Check sheet for the modelled part. Datum: model origin and axes. Units: mm. Give positions to 0.01 mm unless a question says otherwise; leave off trailing zeros. Order: outer loops, then holes, each group sorted by start corner. A loop starts at its lowest first (then second) coordinate and runs counter-clockwise, first axis right, second up.
Item 1: Gauge pin test, flat ends, axial feed: P1, Ø11, axis at x = 22.36, z = 13.1, coming from the -Y side; P2, Ø2, axis at x = -50, z = 9.6, coming from the +Y side; P3, Ø0.9, axis at x = 51, y = 2, coming from the +Z side; P4, Ø0.8, axis at y = 1, z = 22, coming from the -X side. Record the tip position at first contact, or that the pin passes through.
Item 2: Sectioned sample at A-A on x = 40.25. Record the boundary of the cut face in (y, z), and give its area (3 significant figures).
Item 3: Sectioned sample at C-C on z = 13.1. Count the separate pieces of the cut face and the enclosed holes in it, and give its area (4 significant figures).
Item 4: Sectioned sample at B-B on x = -50. Record the boundary of the cut face in (y, z), and give its area (3 significant figures).
Item 5: Material ranges on line 1 along Z through (x, y) = (-4.5, 1.65); line 2 along Z through (x, y) = (40.25, 2.25); line 3 along X through (y, z) = (1.15, 5.25), recorded low to high.
from build123d import *

# Parameters (mm, degrees)
SKETCH_1_R            = 3.5
SKETCH_1_W            = 10
SKETCH_1_H            = 3
EXTRUDE_1_DEPTH       = 3
HOLE_WIZARD_M31_D     = 3.4
HOLE_WIZARD_M31_DEPTH = 10
HOLE_WIZARD_M31_TIP   = 1.021463052
FILLET_1_R            = 0.5
FILLET_2_R            = 0.5


with BuildPart() as part:
    # Эскиз1 → Бобышка-Вытянуть1 (new body)
    with BuildSketch(Plane(origin=(0, 0, 0), x_dir=(1, 0, 0), z_dir=(0, 1, 0))):
        Polygon((-43.75, -21), (43.75, -21), (43.75, -18.5), (56.25, -18.5), (56.25, -15.5), (59.25, -15.5), (59.25, -5.5), (56.25, -5.5), (56.25, 0), (-56.25, 0), (-56.25, -5.5), (-59.25, -5.5), (-59.25, -15.5), (-56.25, -15.5), (-56.25, -18.5), (-43.75, -18.5), align=None)
        with Locations((-40.25, -13.1)):
            Circle(SKETCH_1_R, mode=Mode.SUBTRACT)
        with Locations((-31.305555556, -13.1)):
            Circle(SKETCH_1_R, mode=Mode.SUBTRACT)
        with Locations((-22.361111111, -13.1)):
            Circle(SKETCH_1_R, mode=Mode.SUBTRACT)
        with Locations((-13.416666667, -13.1)):
            Circle(SKETCH_1_R, mode=Mode.SUBTRACT)
        with Locations((-4.472222222, -13.1)):
            Circle(SKETCH_1_R, mode=Mode.SUBTRACT)
        with Locations((4.472222222, -13.1)):
            Circle(SKETCH_1_R, mode=Mode.SUBTRACT)
        with Locations((13.416666667, -13.1)):
            Circle(SKETCH_1_R, mode=Mode.SUBTRACT)
        with Locations((22.361111111, -13.1)):
            Circle(SKETCH_1_R, mode=Mode.SUBTRACT)
        with Locations((31.305555556, -13.1)):
            Circle(SKETCH_1_R, mode=Mode.SUBTRACT)
        with Locations((40.25, -13.1)):
            Circle(SKETCH_1_R, mode=Mode.SUBTRACT)
        with Locations((0, -22.5)):
            Rectangle(SKETCH_1_W, SKETCH_1_H)
    extrude(amount=EXTRUDE_1_DEPTH)

    # Отверстие с зазором M31
    with Locations(Plane(origin=(0, 3, 0), x_dir=(1, 0, 0), z_dir=(0, 1, 0))):
        with Locations((50, -9.6), (-50, -9.6)):
            Hole(HOLE_WIZARD_M31_D / 2, depth=HOLE_WIZARD_M31_DEPTH)
            with Locations((0, 0, -(HOLE_WIZARD_M31_DEPTH + HOLE_WIZARD_M31_TIP / 2))):  # 118° drill point
                Cone(0, HOLE_WIZARD_M31_D / 2, HOLE_WIZARD_M31_TIP, mode=Mode.SUBTRACT)

    # Скругление1
    fillet_1_edges = [part.edges().sort_by_distance(p)[0] for p in [
        (-59.25, 1.5, 15.5),
        (-59.25, 1.5, 5.5),
        (59.25, 1.5, 5.5),
        (59.25, 1.5, 15.5),
    ]]
    fillet(fillet_1_edges, radius=FILLET_1_R)

    # Скругление2
    fillet_2_edges = [part.edges().sort_by_distance(p)[0] for p in [
        (-56.25, 1.5, 18.5),
        (-56.25, 1.5, 0),
        (56.25, 1.5, 0),
        (56.25, 1.5, 18.5),
        (5, 1.5, 24),
        (-5, 1.5, 24),
    ]]
    fillet(fillet_2_edges, radius=FILLET_2_R)


solid = part.part
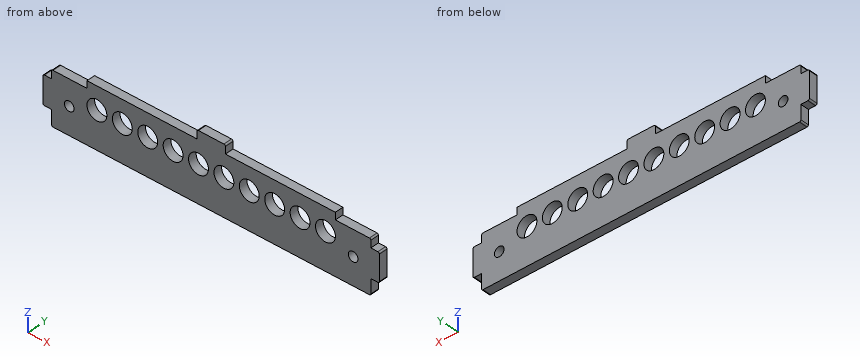
Report:
1. P1: stops at y = 0
1. P2: passes through
1. P3: stops at z = 18.5
1. P4: stops at x = -5
2. outline: (0, 0) - (3, 0) - (3, 9.6) - (0, 9.6) - close; (0, 16.6) - (3, 16.6) - (3, 21) - (0, 21) - close
2. area: 42.0 mm2
3. separate pieces: 11
3. enclosed holes: 0
3. area: 145.5 mm2
4. outline: (0, 0) - (3, 0) - (3, 7.9) - (0, 7.9) - close; (0, 11.3) - (3, 11.3) - (3, 18.5) - (0, 18.5) - close
4. area: 45.3 mm2
5. line 1: z = 0 to 9.6, 16.6 to 24
5. line 2: z = 0 to 9.6, 16.6 to 21
5. line 3: x = -56.25 to 56.25
